Part model, mm, in its own coordinate system. A direction names the side the tool comes from. Coordinates: 2 decimals unless noted, no trailing zeros. Loops run counter-clockwise (first coordinate to the right, second up) from the corner with the lowest first, then second, coordinate; pieces in that order, holes last. Notation, with made-up numbers: (-3, 53.5) -> (43, 53.5) arc R29 cw to (43, 90.5) -> close; hole circle Ø10 at (1.5, 4). An arc over 180 degrees is marked (long way). One line per question, with ' | ' between items. Start each with the question number.
1) Cut at A-A (y = 5.5). List the corners of the cut face in (x, z).
2) Drop flat-ended pins along their axis: pin 1 (2.5 mm diameter, centred on x = 0, z = 0, fed in from +Y); pin 2 (2 mm diameter, centred on y = -2, z = 2.5, fed in from +X); pin 3 (1.5 mm diameter, centred on x = 1, y = 2, fed in from -Z). Give the stop position or say it passes through.
3) 3-axis set-ups, long thin cutter, end or side, ignore diameter. For faces 1 (the face through (-1.115, -16.556, -1.216)), 2 (the face through (-1.3, 20.5, 1.3)), 3 (the face through (0.9, 12.39, 2.86)): which of +Z, -Z, +X, -X, +Y, -Y reach the whole face in a straight line?
4) Cut at B-B (x = -2). List the corners of the cut face in (y, z).
5) Probe L1, parallel to X at y = 16.5, z = 0; L2, parallel to X at y = 13, z = 1.25. List the from-to ranges inside material, lowest first. Write a range as from..to.
6) Two-plate mould, pull along X, no slides. Class faces 4 (the face through (3, 4.5, 1)), 5 (the face through (-1.115, 16.556, -1.216)), 6 (the face through (-3.905, 3.486, -0.867)): released by +X, released by -X, zero draft, split by the parting line, or undercut.
7) Cut at D-D (x = 2.25). List the corners of the cut face in (y, z), plus the area to 3 significant figures.
8) Cut at C-C (y = -15.5). List the corners of the cut face in (x, z), plus the area to 3 significant figures.
from build123d import *

# Parameters (mm, degrees)
BOSS_EXTRUDE1_DEPTH      = 20.5
BOSS_EXTRUDE1_DEPTH_BACK = 20.5
SKETCH1_R                = 3
SKETCH6_R                = 4
BOSS_EXTRUDE2_DEPTH      = 2


with BuildPart() as part:
    # Sketch1 → Boss-Extrude1 (new, two sides: drawn at the far end of the back side and taken through both)
    with BuildSketch(Plane(origin=(0, 0, 0), x_dir=(1, 0, 0), z_dir=(0, 1, 0)).offset(-BOSS_EXTRUDE1_DEPTH_BACK)):
        with Locations(Location((0, 0, 0), (0, 0, 270))):
            Circle(SKETCH1_R)
    extrude(amount=BOSS_EXTRUDE1_DEPTH + BOSS_EXTRUDE1_DEPTH_BACK)

    # Sketch5 → M4x0.7 Tapped Hole1 (revolve, cut)
    with BuildSketch(Plane(origin=(0, 20.5, 0), x_dir=(0, 0, 1), z_dir=(1, 0, 0))):
        Polygon((0, 0), (0, 8.991420021), (1.65, 8), (1.65, 0), align=None)
    m4x0_7_tapped_hole1 = revolve(axis=Axis((0, 26.85, 0), (0, -1, 0)), mode=Mode.SUBTRACT)

    # Sketch6 → Boss-Extrude2 (add)
    with BuildSketch(Plane(origin=(0, 2.5, 0), x_dir=(1, 0, 0), z_dir=(0, 1, 0))):
        with Locations(Location((0, 0, 0), (0, 0, 270))):
            Circle(SKETCH6_R)
    extrude(amount=BOSS_EXTRUDE2_DEPTH)

    # Mirror1: M4x0.7 Tapped Hole1 across plane
    add(m4x0_7_tapped_hole1.mirror(Plane.ZX), mode=Mode.SUBTRACT)


solid = part.part
Reported:
1) outline: circle Ø6 at (0, 0)
2) pin 1: stops at y = 12.26 | pin 2: stops at x = 2.6 | pin 3: stops at z = -3.98
3) face 1: -Y | face 2: +Z, -Z, +X, -X, +Y | face 3: +Y
4) outline: (-20.5, -2.24) -> (2.5, -2.24) -> (2.5, -3.46) -> (4.5, -3.46) -> (4.5, -2.24) -> (20.5, -2.24) -> (20.5, 2.24) -> (4.5, 2.24) -> (4.5, 3.46) -> (2.5, 3.46) -> (2.5, 2.24) -> (-20.5, 2.24) -> close
5) L1: x = -3..-1.65, 1.65..3 | L2: x = -2.73..-1.08, 1.08..2.73
6) face 4: zero draft | face 5: undercut | face 6: split by the parting line
7) outline: (-20.5, -1.98) -> (2.5, -1.98) -> (2.5, -3.31) -> (4.5, -3.31) -> (4.5, -1.98) -> (20.5, -1.98) -> (20.5, 1.98) -> (4.5, 1.98) -> (4.5, 3.31) -> (2.5, 3.31) -> (2.5, 1.98) -> (-20.5, 1.98) -> close | area: 168 mm²
8) outline: circle Ø6 at (0, 0); hole circle Ø3.3 at (0, 0) | area: 19.7 mm²
